Model file for the job. Use its own axes, mm. Face numbers are marked on the shaded views. Round coordinates to 2 decimals unless told otherwise and drop trailing zeros. Write each loop counter-clockwise with the first axis right and the second up, starting at its lowest first coordinate (ties: lowest second). Pieces come first, ordered by that corner, then holes. Notation, with made-up numbers: (52.25, 6) - (66.25, 6) arc R24 ccw to (66.25, 41) - close; hole circle Ø8 at (35.5, 78.25). An arc over 180 degrees is marked (long way). One line per item, written item: value.
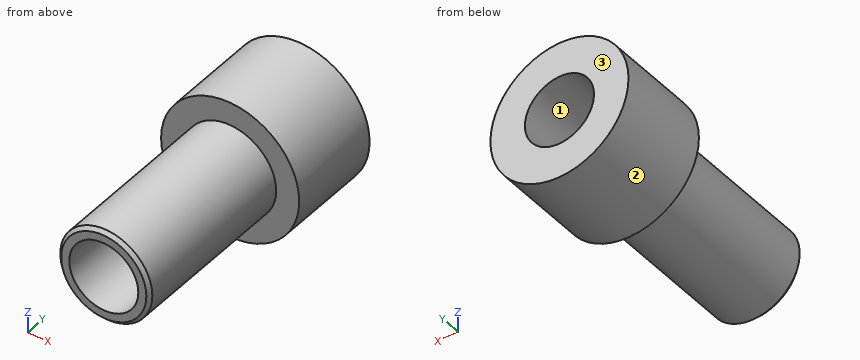
from build123d import *

# Parameters (mm, degrees)
F0_R     = 6
F0_R_2   = 4
F1_DEPTH = 8.3
F0_R_3   = 3
F2_DEPTH = 23.2
F3_SIZE  = 0.3


with BuildPart() as f1:
    # F0 (on Front) → F1 (new body)
    with BuildSketch(Plane.XZ):
        Circle(F0_R)
        Circle(F0_R_2, mode=Mode.SUBTRACT)
    extrude(amount=F1_DEPTH)

    # F0 (on Front) → F2 (join)
    with BuildSketch(Plane.XZ):
        Circle(F0_R_2)
        Circle(F0_R_3, mode=Mode.SUBTRACT)
    extrude(amount=F2_DEPTH)

    # F3
    f3_edges = [f1.edges().sort_by_distance(p)[0] for p in [
        (-4, -23.2, 0),
    ]]
    chamfer(f3_edges, length=F3_SIZE)


solid = f1.part
1. Band-saw the part on C-C on y = -13.5. Write the cut outline in (x, z).
Report:
outline: circle Ø8 at (0, 0); hole circle Ø6 at (0, 0)
2. Mould opens along X. For the marked faces 1, 2 and 3 say: released by +X, released by -X, zero draft, split by the parting line, or undercut.
Report:
face 1: undercut
face 2: split by the parting line
face 3: zero draft
3. Band-saw the part on D-D on x = -4.75. Write the cut outline in (y, z).
Report:
outline: (-8.3, -3.67) - (0, -3.67) - (0, 3.67) - (-8.3, 3.67) - close
4. Band-saw the part on A-A on z = 0. Write the cut outline in (x, y), plus the area to 3 significant figures.
Report:
outline: (-6, -8.3) - (-4, -8.3) - (-4, -22.9) - (-3.7, -23.2) - (-3, -23.2) - (-3, 0) - (-6, 0) - close; (3, -23.2) - (3.7, -23.2) - (4, -22.9) - (4, -8.3) - (6, -8.3) - (6, 0) - (3, 0) - close
area: 79.5 mm²
5. Wall check: probe 1 along Z at (x, y) = (0, -13); probe 2 along Z at (x, y) = (0, -8); probe 3 along Y at (x, z) = (0, -4.5). Give the ranges that are in metal, low to high. Write a range as [from, to].
Report:
probe 1: [-4, -3], [3, 4]
probe 2: [-6, -3], [3, 6]
probe 3: [-8.3, 0]
6. Drop flat-ended pins along their axis: pin 1 (5 mm diameter, centred on y = -18.5, z = -3, fed in from -X); pin 2 (4 mm diameter, centred on y = -18, z = -2.5, fed in from +X); pin 3 (4 mm diameter, centred on x = 3, z = -2.5, fed in from +Y); pin 4 (5 mm diameter, centred on x = 0, z = 0, fed in from -Y). Give the stop position or say it passes through.
Report:
pin 1: x = -3.97
pin 2: x = 3.97
pin 3: y = 0
pin 4: through
7. Band-saw the part on B-B on x = 0. Write the cut outline in (y, z), plus the area to 3 significant figures.
Report:
outline: (-23.2, -3.7) - (-22.9, -4) - (-8.3, -4) - (-8.3, -6) - (0, -6) - (0, -3) - (-23.2, -3) - close; (-23.2, 3) - (0, 3) - (0, 6) - (-8.3, 6) - (-8.3, 4) - (-22.9, 4) - (-23.2, 3.7) - close
area: 79.5 mm²
